```python
from build123d import *

# Parameters (mm, degrees)
SKETCH1_R                                       = 2.6
BOSS_EXTRUDE1_DEPTH                             = 6
SKETCH2_R                                       = 3.25
BOSS_EXTRUDE2_DEPTH                             = 2
SKETCH3_R                                       = 2.5
BOSS_EXTRUDE3_DEPTH                             = 2.7
CSK_FOR_M5_FLAT_HEAD_MACHINE_SCREW1_D           = 5.5
CSK_FOR_M5_FLAT_HEAD_MACHINE_SCREW1_CSINK_D     = 10.4
CSK_FOR_M5_FLAT_HEAD_MACHINE_SCREW1_CSINK_ANGLE = 90
SKETCH7_R                                       = 2.6
BOSS_EXTRUDE5_DEPTH                             = 21


with BuildPart() as part:
    # Sketch1 → Boss-Extrude1 (new body)
    with BuildSketch(Plane(origin=(0, 0, 0), x_dir=(1, 0, 0), z_dir=(0, 1, 0))):
        with BuildLine():
            Line((5.031184409, -3), (0, -3))
            Line((0, -3), (0, -46))
            Line((0, -46), (50, -46))
            Line((50, -46), (50, -3))
            Line((50, -3), (44.968815591, -3))
            ThreePointArc((44.968815591, -3), (25, -7.79226602), (5.031184409, -3))
        make_face()
        with Locations(Location((15, -36, 0), (0, 0, 270))):
            Circle(SKETCH1_R, mode=Mode.SUBTRACT)
        with Locations(Location((35, -36, 0), (0, 0, 270))):
            Circle(SKETCH1_R, mode=Mode.SUBTRACT)
        with Locations(Location((15, -16, 0), (0, 0, 270))):
            Circle(SKETCH1_R, mode=Mode.SUBTRACT)
        with Locations(Location((35, -16, 0), (0, 0, 270))):
            Circle(SKETCH1_R, mode=Mode.SUBTRACT)
    extrude(amount=BOSS_EXTRUDE1_DEPTH)

    # Sketch2 → Boss-Extrude2 (add)
    with BuildSketch(Plane(origin=(0, 6, 0), x_dir=(1, 0, 0), z_dir=(0, 1, 0))):
        with Locations(Location((25, -17.5, 0), (0, 0, 270))):
            Circle(SKETCH2_R)
    extrude(amount=BOSS_EXTRUDE2_DEPTH)

    # Sketch3 → Boss-Extrude3 (add)
    with BuildSketch(Plane(origin=(0, 8, 0), x_dir=(1, 0, 0), z_dir=(0, 1, 0))):
        with Locations(Location((25, -17.5, 0), (0, 0, 90))):
            Circle(SKETCH3_R)
    extrude(amount=BOSS_EXTRUDE3_DEPTH)

    # CSK for M5 Flat Head Machine Screw1 (through all)
    with Locations(Plane(origin=(0, 6, 0), x_dir=(1, 0, 0), z_dir=(0, 1, 0))):
        with Locations((15, -16), (35, -16)):
            CounterSinkHole(CSK_FOR_M5_FLAT_HEAD_MACHINE_SCREW1_D / 2, CSK_FOR_M5_FLAT_HEAD_MACHINE_SCREW1_CSINK_D / 2, counter_sink_angle=CSK_FOR_M5_FLAT_HEAD_MACHINE_SCREW1_CSINK_ANGLE)

    # Sketch7 → Boss-Extrude5 (add)
    with BuildSketch(Plane(origin=(0, 6, 0), x_dir=(1, 0, 0), z_dir=(0, 1, 0))):
        with BuildLine():
            Line((21.039948447, -30.928253487), (0, -30.928253487))
            Line((0, -30.928253487), (0, -46))
            Line((0, -46), (50, -46))
            Line((50, -46), (50, -30.580877922))
            Line((50, -30.580877922), (29.989051292, -30.580877922))
            ThreePointArc((29.989051292, -30.580877922), (25.543026299, -31.489464694), (21.039948447, -30.928253487))
        make_face()
        with Locations(Location((15, -36, 0), (0, 0, 270))):
            Circle(SKETCH7_R, mode=Mode.SUBTRACT)
        with Locations(Location((35, -36, 0), (0, 0, 270))):
            Circle(SKETCH7_R, mode=Mode.SUBTRACT)
    extrude(amount=BOSS_EXTRUDE5_DEPTH)


solid = part.part
```
Read the model definition and answer for the solid it produces. Units are mm, in the model's axes. A direction names the side the tool comes from. Coordinates: 2 decimals unless noted, no trailing zeros. Loops run counter-clockwise (first coordinate to the right, second up) from the corner with the lowest first, then second, coordinate; pieces in that order, holes last.
(1) The part is cut by section A-A (y = 4.25). Determine the outline of the cut face in (x, z).
Solution:
outline: (0, 3) - (5.03, 3) arc R44 cw to (44.97, 3) - (50, 3) - (50, 46) - (0, 46) - close; hole circle Ø6.9 at (15, 16); hole circle Ø5.2 at (15, 36); hole circle Ø6.9 at (35, 16); hole circle Ø5.2 at (35, 36)
(2) A tool of negligible diameter and unlimited length cuts with its end or side. For faces 1 (the face through (23.022, 6.986, 14.921)), 2 (the face through (3, 3, 3)), 3 (the face through (25.29, 2.96, 7.79)), 4 (the face through (25, 10.7, 18)), 5 (the face through (11, 16, 30.928)), from which of +Z, -Z, +X, -X, +Y, -Y can it reach the whole face along a straight path? Write none if from no direction.
Solution:
face 1: +Y
face 2: -Z, +X, -X, +Y, -Y
face 3: -Z, +Y, -Y
face 4: -Z, +X, -X, +Y
face 5: -Z, -X, +Y
(3) The part is cut by section D-D (x = 15). Determine the outline of the cut face in (y, z).
Solution:
outline: (0, 6.64) - (6, 6.64) - (6, 10.8) - (3.55, 13.25) - (0, 13.25) - close; (0, 18.75) - (3.55, 18.75) - (6, 21.2) - (6, 30.93) - (27, 30.93) - (27, 33.4) - (0, 33.4) - close; (0, 38.6) - (27, 38.6) - (27, 46) - (0, 46) - close
(4) Consider line 1 along X through (y, z) = (16.75, 36); line 2 along X through (y, z) = (1.7, 16); line 3 along Z through (x, y) = (31, 10.5). Determine where each line is inside the solid, lowest interval first.
Solution:
line 1: x = 0 to 12.4, 17.6 to 32.4, 37.6 to 50
line 2: x = 0 to 12.25, 17.75 to 32.25, 37.75 to 50
line 3: z = 30.58 to 46
(5) Flat-ended cylindrical pins translate along their axes: pin 1 Ø3 at (x, z) = (35, 36) entering from -Y; pin 2 Ø6.5 at (x, z) = (35, 16) entering from +Y; pin 3 Ø6 at (x, y) = (7, 18) entering from -Z; pin 4 Ø1.5 at (x, z) = (10.5, 21) entering from +Y. Find the tip coordinate at first contact, or state that the pin passes through.
Solution:
pin 1: passes through
pin 2: stops at y = 4.05
pin 3: stops at z = 30.93
pin 4: stops at y = 6
(6) The mould has two halves that part along X. Classify faces 6 (the face through (25, 13, 46)), 7 (the face through (23, 9, 19)), 8 (the face through (13.418, 13.311, 33.937)): released by +X, released by -X, zero draft, split by the parting line, or undercut.
Solution:
face 6: zero draft
face 7: split by the parting line
face 8: undercut
(7) The part is cut by section C-C (z = 36). Determine the outline of the cut face in (x, y), and give its area (3 significant figures).
Solution:
outline: (0, 0) - (12.4, 0) - (12.4, 27) - (0, 27) - close; (17.6, 0) - (32.4, 0) - (32.4, 27) - (17.6, 27) - close; (37.6, 0) - (50, 0) - (50, 27) - (37.6, 27) - close
area: 1,070 mm2
(8) The part is cut by section B-B (y = 18.25). Determine the outline of the cut face in (x, z).
Solution:
outline: (0, 30.93) - (21.04, 30.93) arc R14 cw to (29.99, 30.58) - (50, 30.58) - (50, 46) - (0, 46) - close; hole circle Ø5.2 at (15, 36); hole circle Ø5.2 at (35, 36)
